Check sheet for the modelled part. Datum: model origin and axes. Units: mm. Coordinates: 2 decimals unless noted, no trailing zeros. Loops run counter-clockwise (first coordinate to the right, second up) from the corner with the lowest first, then second, coordinate; pieces in that order, holes last. Notation, with made-up numbers: M -9.5,54 L 12.5,54 A25 ccw 12.5,78 Z; hole C -37.75,57 d8. An arc over 180 degrees is marked long. Answer in a Markdown table with one row per item. Add a question column.
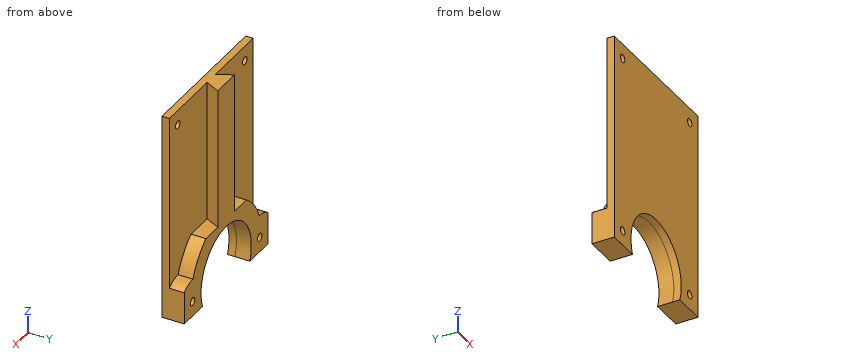
```python
from build123d import *

# Parameters (mm, degrees)
SKETCH1_W                    = 127
SKETCH1_H                    = 177.8
BOSS_EXTRUDE1_DEPTH          = 6.35
H_0_266_DIAMETER_HOLE1_D     = 6.7564
H_0_266_DIAMETER_HOLE1_DEPTH = 16.51
H_0_266_DIAMETER_HOLE1_TIP   = 2.029827343
SKETCH4_R                    = 38.1
CUT_EXTRUDE1_DEPTH           = 6.35
SKETCH5_R                    = 3.3782
BOSS_EXTRUDE2_DEPTH          = 12.7
BOSS_EXTRUDE3_DEPTH          = 121.666
SKETCH7_W                    = 27.292671225
SKETCH7_H                    = 12.7
CUT_EXTRUDE2_DEPTH           = 120.65


with BuildPart() as part:
    # Sketch1 → Boss-Extrude1 (new body)
    with BuildSketch(Plane(origin=(0, 0, 0), x_dir=(1, 0, 0), z_dir=(0, 1, 0))):
        Rectangle(SKETCH1_W, SKETCH1_H)
    extrude(amount=BOSS_EXTRUDE1_DEPTH)

    # H (0.266) Diameter Hole1
    with Locations(Plane(origin=(0, 6.35, 0), x_dir=(1, 0, 0), z_dir=(0, 1, 0))):
        with Locations((-50.8, 76.2), (50.8, -76.2), (50.8, 76.2), (-50.8, -76.2)):
            Hole(H_0_266_DIAMETER_HOLE1_D / 2, depth=H_0_266_DIAMETER_HOLE1_DEPTH)
            with Locations((0, 0, -(H_0_266_DIAMETER_HOLE1_DEPTH + H_0_266_DIAMETER_HOLE1_TIP / 2))):  # 118° drill point
                Cone(0, H_0_266_DIAMETER_HOLE1_D / 2, H_0_266_DIAMETER_HOLE1_TIP, mode=Mode.SUBTRACT)

    # Sketch4 → Cut-Extrude1 (cut)
    with BuildSketch(Plane(origin=(0, 6.35, 0), x_dir=(1, 0, 0), z_dir=(0, 1, 0))):
        with Locations((0, 76.2)):
            Circle(SKETCH4_R)
    extrude(amount=-CUT_EXTRUDE1_DEPTH, mode=Mode.SUBTRACT)

    # Sketch5 → Boss-Extrude2 (add)
    with BuildSketch(Plane(origin=(0, 6.35, 0), x_dir=(1, 0, 0), z_dir=(0, 1, 0))):
        with BuildLine():
            Line((-35.921024484, 88.9), (-63.5, 88.9))
            Line((-63.5, 88.9), (-63.5, 61.321024484))
            ThreePointArc((-63.5, 61.321024484), (-57.336478943, 57.762311549), (-50.307743234, 56.644141653))
            ThreePointArc((-50.307743234, 56.644141653), (0, 22.225), (50.307743234, 56.644141653))
            ThreePointArc((50.307743234, 56.644141653), (57.336478943, 57.762311549), (63.5, 61.321024484))
            Line((63.5, 61.321024484), (63.5, 88.9))
            Line((63.5, 88.9), (35.921024484, 88.9))
            ThreePointArc((35.921024484, 88.9), (0, 38.1), (-35.921024484, 88.9))
        make_face()
        with Locations(Location((50.8, 76.2, 0), (0, 0, 270))):
            Circle(SKETCH5_R, mode=Mode.SUBTRACT)
        with Locations(Location((-50.8, 76.2, 0), (0, 0, 270))):
            Circle(SKETCH5_R, mode=Mode.SUBTRACT)
    extrude(amount=BOSS_EXTRUDE2_DEPTH)

    # Sketch6 → Boss-Extrude3 (add)
    with BuildSketch(Plane.XY.offset(88.9)):
        Polygon((-12.7, 19.05), (-6.35, 6.35), (6.35, 6.35), (12.7, 19.05), align=None)
    extrude(amount=-BOSS_EXTRUDE3_DEPTH)

    # Sketch7 → Cut-Extrude2 (cut)
    with BuildSketch(Plane.XY.offset(88.9)):
        with Locations((-36.661407622, 12.7)):
            Rectangle(SKETCH7_W, SKETCH7_H)
        Polygon((-23.015072009, 19.05), (-23.015072009, 6.35), (-6.35, 6.35), (-12.7, 19.05), align=None)
        Polygon((6.35, 6.35), (23.015072009, 6.35), (23.015072009, 19.05), (12.7, 19.05), align=None)
        with Locations((36.661407622, 12.7)):
            Rectangle(SKETCH7_W, SKETCH7_H)
    extrude(amount=-CUT_EXTRUDE2_DEPTH, mode=Mode.SUBTRACT)


solid = part.part
```
Q1. Thickness scan on L1, parallel to Z at x = -50.8, y = 4; L2, parallel to X at y = 12, z = -76.2; L3, parallel to X at y = 4, z = 76.2. Record the ranges inside material, lowest first.
Q2. Cross-section at D-D (x = 25). Record the cut outline in (y, z).
Q3. Go/stop test with flat-tipped pins: pin 1 (5.5 mm diameter, centred on x = -50.8, z = 76.2, fed in from +Y); pin 2 (10 mm diameter, centred on x = 15, y = 6.5, fed in from -Z); pin 3 (17 mm diameter, centred on x = -46, z = 28, fed in from +Y); pin 4 (4 mm diameter, centred on x = -15, y = 14, fed in from +Z). Record where each tip stops, or that it passes through.
Q4. Cross-section at C-C (z = -76.2). Record the cut outline in (x, y).
Q5. Cross-section at B-B (y = 4.25). Record the cut outline in (x, z), plus the area to 3 significant figures.
Q6. Cross-section at A-A (z = 76.2). Record the cut outline in (x, y), plus the area to 3 significant figures.
Answer key:
| question | item | result |
|---|---|---|
| 1 | L1 | -88.9 to -79.58, -72.82 to 72.82, 79.58 to 88.9 |
| 1 | L2 | -63.5 to -54.18, -47.42 to -38.1, 38.1 to 47.42, 54.18 to 63.5 |
| 1 | L3 | -63.5 to -54.18, -47.42 to 47.42, 54.18 to 63.5 |
| 2 | outline | M 0,-47.45 L 19.05,-47.45 L 19.05,-31.75 L 6.35,-31.75 L 6.35,88.9 L 0,88.9 Z |
| 3 | pin 1 | through |
| 3 | pin 2 | z = -43.77 |
| 3 | pin 3 | y = 6.35 |
| 3 | pin 4 | z = -31.75 |
| 4 | outline | M -63.5,0 L -54.18,0 L -54.18,19.05 L -63.5,19.05 Z; M -47.42,0 L -38.1,0 L -38.1,19.05 L -47.42,19.05 Z; M 38.1,0 L 47.42,0 L 47.42,19.05 L 38.1,19.05 Z; M 54.18,0 L 63.5,0 L 63.5,19.05 L 54.18,19.05 Z |
| 5 | outline | M -63.5,-88.9 L -35.92,-88.9 A38.1 cw long 35.92,-88.9 L 63.5,-88.9 L 63.5,88.9 L -63.5,88.9 Z; hole C -50.8,-76.2 d6.76; hole C -50.8,76.2 d6.76; hole C 50.8,-76.2 d6.76; hole C 50.8,76.2 d6.76 |
| 5 | area | 19,200 mm^2 |
| 6 | outline | M -63.5,0 L -54.18,0 L -54.18,6.35 L -63.5,6.35 Z; M -47.42,0 L 47.42,0 L 47.42,6.35 L 6.35,6.35 L 12.7,19.05 L -12.7,19.05 L -6.35,6.35 L -47.42,6.35 Z; M 54.18,0 L 63.5,0 L 63.5,6.35 L 54.18,6.35 Z |
| 6 | area | 963 mm^2 |
